For this review, use the dimensioned drawing (mm, ordinates from the lowest corner) and the shaded views. A direction names the side the tool comes from. Round coordinates to 2 decimals unless told otherwise and drop trailing zeros. Order: outer loops, then holes, each group sorted by start corner. A loop starts at its lowest first (then second) coordinate and runs counter-clockwise, first axis right, second up. Notation, with made-up numbers: (55.25, 7.25) - (80.25, 7.25) arc R22 cw to (80.25, 15.25) - close; hole circle Ø8 at (19.5, 6). An arc over 180 degrees is marked (long way). Write each question's results on one line, items separated by ' | '. Start each with the question number.
(1) Take a section at A-A, the plane x = 19. Give the boundary of the cut face in (y, z).
(2) Draft analysis for pull direction Z (two halves, no side actions). For the marked faces 4, 5 and 6, state which applies: pulls with the +Z half, pulls with the -Z half, needs draft (parallel to the pull), parting line crosses it, or undercut.
(3) Insertion check: pin 1 Ø1.5 at (x, z) = (15, 13) entering from -Y; pin 2 Ø4 at (x, z) = (30, 12.5) entering from +Y. Each pin has a flat end and moves straight along its axis. Give the tip position at first contact, or say it passes through.
(4) Take a section at B-B, the plane z = 12. Give the boundary of the cut face in (x, y).
(5) Take a section at C-C, the plane y = 18.75. Give the boundary of the cut face in (x, z), plus the area to 3 significant figures.
(6) For L1, parallel to Z at x = 19, y = 8.5; L2, parallel to X at y = 7.15, z = 12; L3, parallel to X at y = 10.5, z = 19, list the stretches that pass through material, from the lowest coordinate up. Write a range as from..to.
(7) Take a section at D-D, the plane x = 33. Give the boundary of the cut face in (y, z), plus the area to 3 significant figures.
(8) For the marked faces 1, 2 and 3, list the 3-axis set-ups (+Z, -Z, +X, -X, +Y, -Y) from which the entire face can be reached by the end or side of a thin tool; tool diameter is ignored.
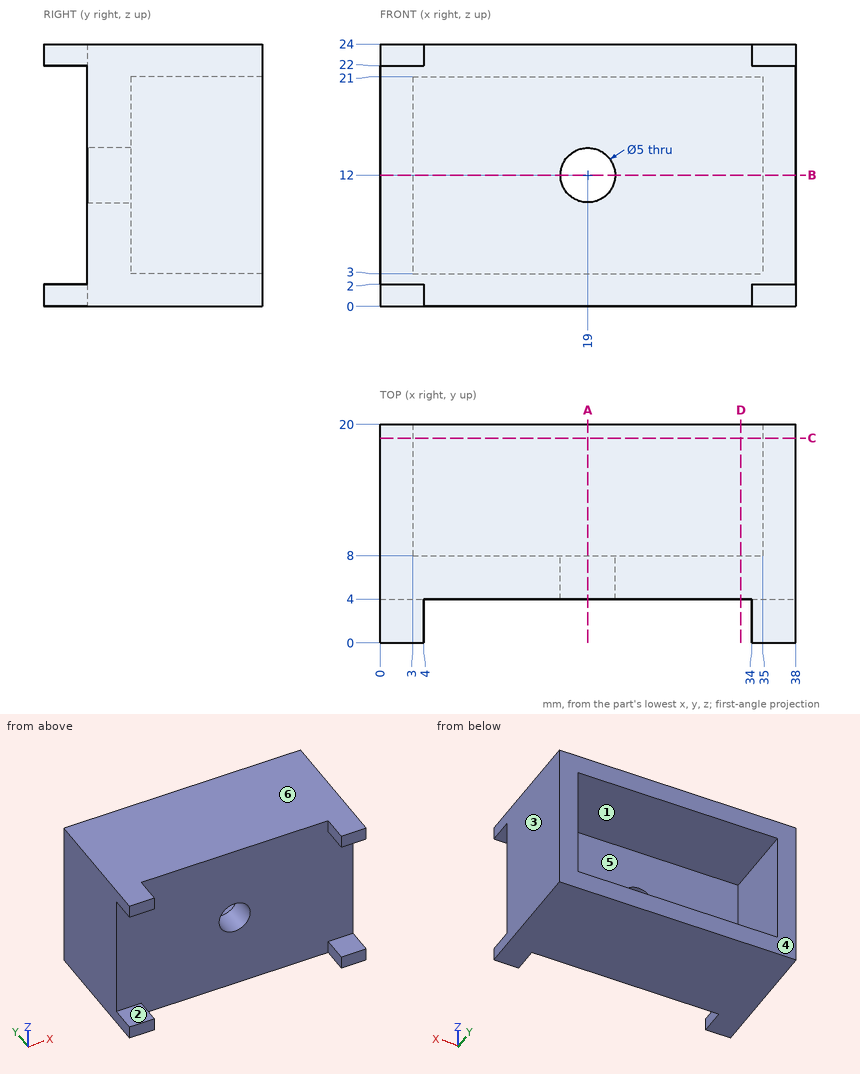
Results below:
1) outline: (4, 0) - (20, 0) - (20, 3) - (8, 3) - (8, 9.5) - (4, 9.5) - close; (4, 14.5) - (8, 14.5) - (8, 21) - (20, 21) - (20, 24) - (4, 24) - close
2) face 4: needs draft | face 5: undercut | face 6: pulls with the +Z half
3) pin 1: stops at y = 4 | pin 2: stops at y = 8
4) outline: (0, 4) - (16.5, 4) - (16.5, 8) - (3, 8) - (3, 20) - (0, 20) - close; (21.5, 4) - (38, 4) - (38, 20) - (35, 20) - (35, 8) - (21.5, 8) - close
5) outline: (0, 0) - (38, 0) - (38, 24) - (0, 24) - close; hole (3, 3) - (35, 3) - (35, 21) - (3, 21) - close | area: 336 mm^2
6) L1: z = 0..3, 21..24 | L2: x = 0..16.5, 21.5..38 | L3: x = 0..3, 35..38
7) outline: (4, 0) - (20, 0) - (20, 3) - (8, 3) - (8, 21) - (20, 21) - (20, 24) - (4, 24) - close | area: 168 mm^2
8) face 1: +Y | face 2: +X, -X, -Y | face 3: +Z, -Z, +X, +Y, -Y
